Can you work these out from the model? Positions are in its coordinate system, mm. A direction names the side the tool comes from. Give positions to 0.01 mm unless a question says otherwise; leave off trailing zeros. Write each loop counter-clockwise with the first axis right and the second up, starting at its lowest first coordinate (ties: lowest second). Pieces come first, ordered by that corner, then holes.
from build123d import *

# Parameters (mm, degrees)
SKETCH_W        = 55
SKETCH_H        = 56
PAD_DEPTH       = 12
SKETCH012_W     = 52.6
SKETCH012_H     = 53.6
POCKET_DEPTH    = 10.8
SKETCH013_W     = 26
SKETCH013_H     = 30
PAD010_DEPTH    = 5
SKETCH014_W     = 18
SKETCH014_H     = 6
POCKET001_DEPTH = 5
SKETCH015_W     = 18
SKETCH015_H     = 22
POCKET002_DEPTH = 4
SKETCH016_W     = 19
SKETCH016_H     = 7.4
POCKET003_DEPTH = 5
SKETCH017_R     = 0.9
POCKET004_DEPTH = 4


with BuildPart() as part:
    # Sketch → Pad (new body)
    with BuildSketch(Plane.XY):
        Rectangle(SKETCH_W, SKETCH_H)
    extrude(amount=PAD_DEPTH)

    # Sketch012 (on Face6 of Pad) → Pocket (cut)
    with BuildSketch(Plane.XY.offset(12)):
        Rectangle(SKETCH012_W, SKETCH012_H)
    extrude(amount=-POCKET_DEPTH, mode=Mode.SUBTRACT)

    # Sketch013 (on Face11 of Pocket) → Pad010 (join)
    with BuildSketch(Plane.XY.offset(1.2)):
        with Locations((0, -11.8)):
            Rectangle(SKETCH013_W, SKETCH013_H)
    extrude(amount=PAD010_DEPTH)

    # Sketch014 (on Face13 of Pad010) → Pocket001 (cut)
    with BuildSketch(Plane.XY.offset(6.2)):
        with Locations((0, -20.8)):
            Rectangle(SKETCH014_W, SKETCH014_H)
    extrude(amount=-POCKET001_DEPTH, mode=Mode.SUBTRACT)

    # Sketch015 (on Face13 of Pocket001) → Pocket002 (cut)
    with BuildSketch(Plane.XY.offset(6.2)):
        with Locations((0, -6.8)):
            Rectangle(SKETCH015_W, SKETCH015_H)
    extrude(amount=-POCKET002_DEPTH, mode=Mode.SUBTRACT)

    # Sketch016 (on Face6 of Pocket002) → Pocket003 (cut)
    with BuildSketch(Plane.XZ.offset(28)):
        with Locations((0, 7.2)):
            Rectangle(SKETCH016_W, SKETCH016_H)
    extrude(amount=-POCKET003_DEPTH, mode=Mode.SUBTRACT)

    # Sketch017 (on DatumPlane) → Pocket004 (cut)
    with BuildSketch(Plane.XY.offset(6.2)):
        with Locations((-11, -12)):
            Circle(SKETCH017_R)
        with Locations((11, -12)):
            Circle(SKETCH017_R)
    extrude(amount=-POCKET004_DEPTH, mode=Mode.SUBTRACT)


solid = part.part
(1) For faces 1 (the face through (0, -26, 3.5)), 2 (the face through (0, 28, 6)), 3 (the face through (12.3, -11.6, 6.2)), which set-ups out of +Z, -Z, +X, -X, +Y, -Y let a thin tool reach every point of the face, with its end or its side?
Returned:
face 1: -Y
face 2: +Z, -Z, +X, -X, +Y
face 3: +Z
(2) Imagine slicing it at B-B, the plane y = 10. Write out the boundary of the cut face in (x, z).
Returned:
outline: (-27.5, 0) - (27.5, 0) - (27.5, 12) - (26.3, 12) - (26.3, 1.2) - (-26.3, 1.2) - (-26.3, 12) - (-27.5, 12) - close
(3) Imagine slicing it at D-D, the plane z = 7.75. Write out the boundary of the cut face in (x, y), plus the area to 3 significant figures.
Returned:
outline: (-27.5, -28) - (-9.5, -28) - (-9.5, -26.8) - (-26.3, -26.8) - (-26.3, 26.8) - (26.3, 26.8) - (26.3, -26.8) - (9.5, -26.8) - (9.5, -28) - (27.5, -28) - (27.5, 28) - (-27.5, 28) - close
area: 238 mm2
(4) If we mould it in two halves opening along Z, with no side actions, what happens to faces 4 (the face through (26.3, 0, 7)), 5 (the face through (0, -27, 10.9)), 6 (the face through (0, -7, 2.2)), 7 (the face through (0, 0, 0))? For each: +Z half, -Z half, draft (parallel to the pull), parting line (faces both ways), or undercut.
Returned:
face 4: draft
face 5: undercut
face 6: +Z half
face 7: -Z half
(5) If I drill on L1, parallel to Y at x = 11, z = 4.45; L2, parallel to X at y = 3, z = 2; L3, parallel to Y at x = -25, z = 7, over which ranges is the centre line in solid material (lowest first)?
Returned:
L1: y = -28 to -12.9, -11.1 to 3.2, 26.8 to 28
L2: x = -27.5 to -26.3, -13 to 13, 26.3 to 27.5
L3: y = -28 to -26.8, 26.8 to 28
(6) Will these pins go through, and if not, where does the flat tip stop? P1, Ø14.5, axis at x = -1.5, y = -8.5, coming from the +Z side; P2, Ø6, axis at x = 14, y = -17.5, coming from the -Z side; P3, Ø0.9, axis at x = -11.5, y = -12, coming from the +Z side; P4, Ø2, axis at x = -1, y = 6, coming from the +Z side.
Returned:
P1: stops at z = 2.2
P2: stops at z = 0
P3: stops at z = 6.2
P4: stops at z = 1.2
(7) Imagine slicing it at C-C, the plane x = 22.5. Write out the boundary of the cut face in (y, z).
Returned:
outline: (-28, 0) - (28, 0) - (28, 12) - (26.8, 12) - (26.8, 1.2) - (-26.8, 1.2) - (-26.8, 12) - (-28, 12) - close
(8) Imagine slicing it at A-A, the plane x = 3.5. Write out the boundary of the cut face in (y, z), plus the area to 3 significant figures.
Returned:
outline: (-28, 0) - (28, 0) - (28, 12) - (26.8, 12) - (26.8, 1.2) - (3.2, 1.2) - (3.2, 2.2) - (-17.8, 2.2) - (-17.8, 1.2) - (-23.8, 1.2) - (-23.8, 3.5) - (-28, 3.5) - close; (-28, 10.9) - (-26.8, 10.9) - (-26.8, 12) - (-28, 12) - close
area: 112 mm2
